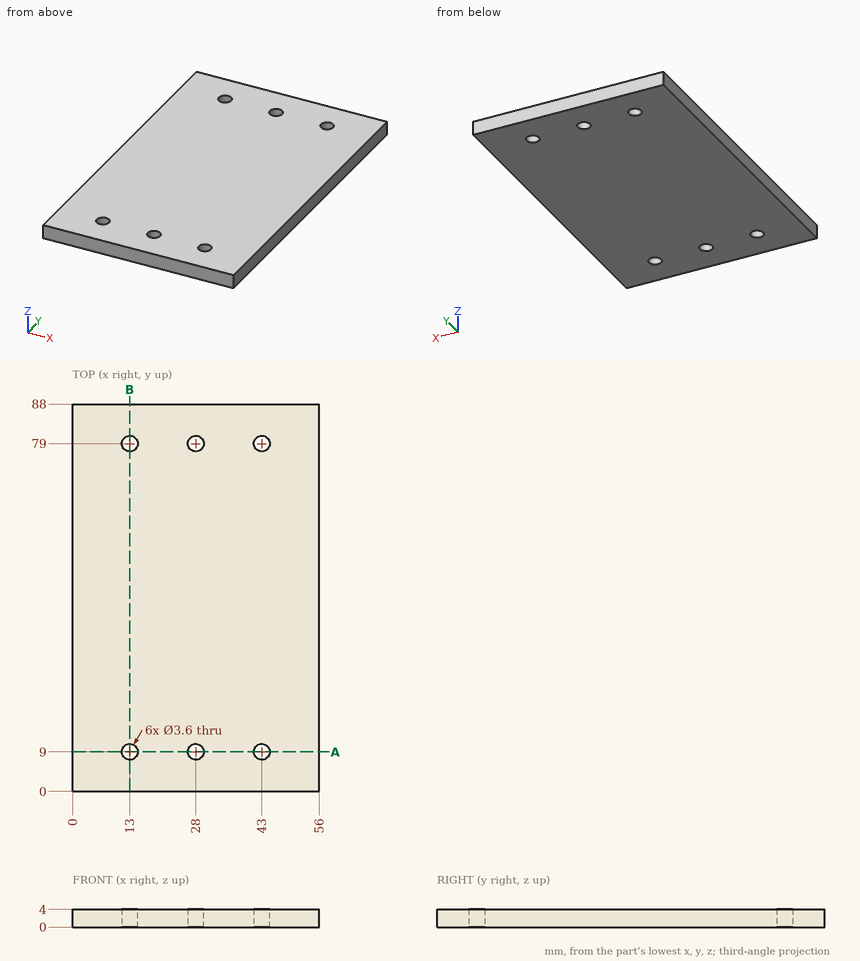
Job drawing, mm, ordinate dimensions from the low corner. One solid piece. Give positions to 0.01 mm unless a question says otherwise; leave off trailing zeros. Write each loop counter-clockwise with the first axis right and the second up, starting at its lowest first coordinate (ties: lowest second). Pieces come first, ordered by that corner, then holes. Notation, with made-up numbers: M 85.25,69 L 92.25,69 A12 cw 92.25,85 Z; hole C 57.25,-24 d11. An arc over 180 degrees is marked long. One line per item, written item: value. Start each with the question number.
Q1. Saw through at B-B, the plane x = 13. Write the cut outline in (y, z).
Q2. Probe probe 1 along X at (y, z) = (79, 1.1); probe 2 along Y at (x, z) = (28, 3.5); probe 3 along X at (y, z) = (7.5, 1.25). List the from-to ranges inside material, lowest first. Write a range as [from, to].
Q3. Saw through at A-A, the plane y = 9. Write the cut outline in (x, z), plus the area to 3 significant figures.
Output values:
1. outline: M 0,0 L 7.2,0 L 7.2,4 L 0,4 Z; M 10.8,0 L 77.2,0 L 77.2,4 L 10.8,4 Z; M 80.8,0 L 88,0 L 88,4 L 80.8,4 Z
2. probe 1: x = [0, 11.2], [14.8, 26.2], [29.8, 41.2], [44.8, 56]
2. probe 2: y = [0, 7.2], [10.8, 77.2], [80.8, 88]
2. probe 3: x = [0, 12.01], [13.99, 27.01], [28.99, 42.01], [43.99, 56]
3. outline: M 0,0 L 11.2,0 L 11.2,4 L 0,4 Z; M 14.8,0 L 26.2,0 L 26.2,4 L 14.8,4 Z; M 29.8,0 L 41.2,0 L 41.2,4 L 29.8,4 Z; M 44.8,0 L 56,0 L 56,4 L 44.8,4 Z
3. area: 181 mm²
